from build123d import *

# Parameters (mm, degrees)
SKETCH1_W            = 15.8
SKETCH1_H            = 3.2
BOSS_EXTRUDE1_DEPTH  = 7.8
SKETCH2_R            = 2.4
BOSS_EXTRUDE2_DEPTH  = 1.6
LPATTERN1_COUNT      = 2
LPATTERN1_PITCH      = 8
LPATTERN1_COUNT_DIR2 = 6
LPATTERN1_PITCH_DIR2 = 8
SHELL1_T             = -1.2
SKETCH3_R            = 1.5
SKETCH3_R_2          = 0.6
BOSS_EXTRUDE3_DEPTH  = 1.8
SKETCH4_W            = 15.8
SKETCH4_H            = 7.8
BOSS_EXTRUDE4_DEPTH  = 1.5
SKETCH5_R            = 2.4
SKETCH5_R_2          = 1.55
BOSS_EXTRUDE5_DEPTH  = 1.6
LPATTERN2_COUNT      = 2
LPATTERN2_PITCH      = 8


with BuildPart() as part:
    # Sketch1 → Boss-Extrude1 (new body)
    with BuildSketch(Plane.XY):
        with Locations((7.9, 1.6)):
            Rectangle(SKETCH1_W, SKETCH1_H)
    extrude(amount=-BOSS_EXTRUDE1_DEPTH)

    # Sketch2 → Boss-Extrude2 (add)
    with BuildSketch(Plane(origin=(0, 3.2, 0), x_dir=(1, 0, 0), z_dir=(0, 1, 0))):
        with Locations(Location((3.9, 3.9, 0), (0, 0, 270))):
            Circle(SKETCH2_R)
    boss_extrude2 = extrude(amount=BOSS_EXTRUDE2_DEPTH)

    # LPattern1: Boss-Extrude2 2 × 6, 10 skipped
    with Locations(*[(j * LPATTERN1_PITCH_DIR2, 0, i * LPATTERN1_PITCH) for i in range(LPATTERN1_COUNT) for j in range(LPATTERN1_COUNT_DIR2) if (i, j) not in ((0, 0), (0, 2), (0, 3), (0, 4), (0, 5), (1, 0), (1, 1), (1, 2), (1, 3), (1, 4), (1, 5))]):
        add(boss_extrude2)

    # Shell1
    shell1_openings = [part.faces().sort_by_distance(p)[0] for p in [
        (7.9, 0, -3.9),
    ]]
    offset(amount=SHELL1_T, openings=shell1_openings, kind=Kind.INTERSECTION)

    # Sketch3 → Boss-Extrude3 (add)
    with BuildSketch(Plane.XZ.offset(-2)):
        with Locations(Location((7.9, -3.9, 0), (0, 0, 90))):
            Circle(SKETCH3_R)
        with Locations(Location((7.9, -3.9, 0), (0, 0, 270))):
            Circle(SKETCH3_R_2, mode=Mode.SUBTRACT)
    extrude(amount=BOSS_EXTRUDE3_DEPTH)

    # Sketch4 → Boss-Extrude4 (add)
    with BuildSketch(Plane(origin=(0, 0, -7.8), x_dir=(-1, 0, 0), z_dir=(0, 0, -1))):
        with Locations((-7.9, -0.7)):
            Rectangle(SKETCH4_W, SKETCH4_H)
    extrude(amount=BOSS_EXTRUDE4_DEPTH)

    # Sketch5 → Boss-Extrude5 (add)
    with BuildSketch(Plane(origin=(0, 0, -9.3), x_dir=(-1, 0, 0), z_dir=(0, 0, -1))):
        with Locations((-3.9, -0.7)):
            Circle(SKETCH5_R)
        with Locations((-3.9, -0.7)):
            Circle(SKETCH5_R_2, mode=Mode.SUBTRACT)
    boss_extrude5 = extrude(amount=BOSS_EXTRUDE5_DEPTH)

    # LPattern2: Boss-Extrude5 ×2
    with Locations(*[(i * LPATTERN2_PITCH, 0, 0) for i in range(1, LPATTERN2_COUNT)]):
        add(boss_extrude5)


solid = part.part
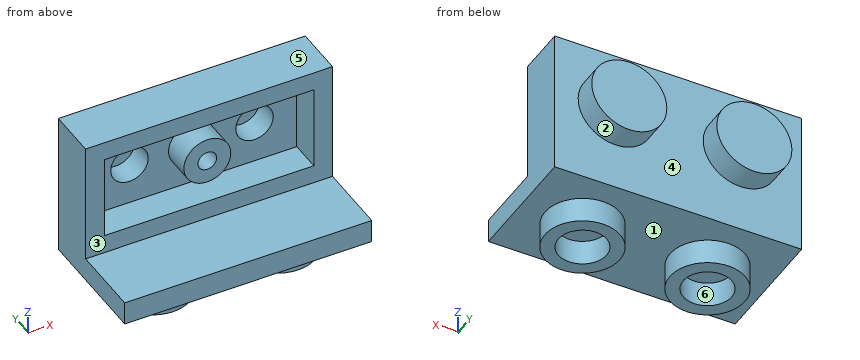
For this review, take the finished solid that the model builds, in its own axes (mm). Face numbers are marked on the shaded views. A direction names the side the tool comes from. Round coordinates to 2 decimals unless told otherwise and drop trailing zeros. Write each loop counter-clockwise with the first axis right and the second up, starting at its lowest first coordinate (ties: lowest second). Pieces come first, ordered by that corner, then holes. Notation, with made-up numbers: (-28.75, 4.25) - (2.25, 4.25) arc R32 ccw to (2.25, 37.25) - close; hole circle Ø1 at (51.25, 54). An arc over 180 degrees is marked (long way). Write item = value, one per line. Start each with the question number.
1. Consider section A-A on y = 0.5. State the section outline as (x, z) points, plus the area to 3 significant figures.
2. Consider section B-B on x = 7.9. State the section outline as (y, z) points, plus the area to 3 significant figures.
3. Draft analysis for pull direction Y (two halves, no side actions). For the marked faces 4, 5 and 6, state which applies: released by +Y, released by -Y, zero draft, split by the parting line, or undercut.
4. Consider section C-C on y = 3. State the section outline as (x, z) points.
5. For the marked faces 1, 2 and 3, list the 3-axis set-ups (+Z, -Z, +X, -X, +Y, -Y) from which the entire face can be reached by the end or side of a thin tool; tool diameter is ignored.
6. For pin 1 Ø5 at (x, y) = (5, 2) entering from +Z; pin 2 Ø0.9 at (x, z) = (7.5, -3.5) entering from -Y; pin 3 Ø4.5 at (x, z) = (10, -4.5) entering from -Y; pin 4 Ø0.7 at (x, z) = (11.5, -4) entering from -Y, all flat-tipped, find the tip position at first contact; note any pin that passes through.
7. Wall thickness on L1, parallel to X at y = 2.7, z = -3.9; L2, parallel to X at y = 3.25, z = -3.9; L3, parallel to Z at x = 11.9, y = 2.9: over which ranges is each line inside the solid? List them lowest first.
Evaluation:
q1.outline = (0, -9.3) - (1.82, -9.3) - (1.82, -10.9) - (2.92, -10.9) - (2.92, -9.3) - (4.88, -9.3) - (4.88, -10.9) - (5.98, -10.9) - (5.98, -9.3) - (9.82, -9.3) - (9.82, -10.9) - (10.92, -10.9) - (10.92, -9.3) - (12.88, -9.3) - (12.88, -10.9) - (13.98, -10.9) - (13.98, -9.3) - (15.8, -9.3) - (15.8, 0) - (0, 0) - close; circle Ø3 at (7.9, -3.9); hole (1.2, -6.6) - (14.6, -6.6) - (14.6, -1.2) - (1.2, -1.2) - close; hole circle Ø1.2 at (7.9, -3.9)
q1.area = 87.5 mm2
q2.outline = (-4.6, -9.3) - (3.2, -9.3) - (3.2, 0) - (0, 0) - (0, -1.2) - (2, -1.2) - (2, -2.4) - (0.2, -2.4) - (0.2, -3.3) - (2, -3.3) - (2, -4.5) - (0.2, -4.5) - (0.2, -5.4) - (2, -5.4) - (2, -6.6) - (0, -6.6) - (0, -7.8) - (-4.6, -7.8) - close
q2.area = 29.1 mm2
q3.face_4 = released by +Y
q3.face_5 = zero draft
q3.face_6 = undercut
q4.outline = (0, -9.3) - (15.8, -9.3) - (15.8, 0) - (0, 0) - close; hole circle Ø2.4 at (3.9, -3.9); hole circle Ø2.4 at (11.9, -3.9)
q5.face_1 = -Z
q5.face_2 = +Y
q5.face_3 = +Z, +X, -X, -Y
q6.pin_1 = 0
q6.pin_2 = 0.2
q6.pin_3 = 0
q6.pin_4 = 3.6
q7.L1 = 0 to 2.7, 5.1 to 10.7, 13.1 to 15.8
q7.L2 = 1.5 to 2.7, 5.1 to 6.3, 9.5 to 10.7, 13.1 to 14.3
q7.L3 = -9.3 to -5.1, -2.7 to 0
